Autodesk Inventor part; units mm, degrees
ref_plane "YZ Plane" through (0, 0, 0) normal (1, 0, 0) x (0, 1, 0)
ref_plane "XZ Plane" through (0, 0, 0) normal (0, 1, 0) x (-1, 0, 0)
ref_plane "XY Plane" through (0, 0, 0) normal (0, 0, 1) x (1, 0, 0)
sketch "Sketch2" plane through (0, 0, 0) normal (0, 0, 1) x (1, 0, 0)
  line L0 (150, -175) -> (-150, -175)
  line L1 (-150, -175) -> (-150, 175)
  line L2 (-150, 175) -> (150, 175)
  line L3 (150, 175) -> (150, -175)
  line L4 (150, -175) -> (-150, 175) construction
  line L5 (-150, -175) -> (150, 175) construction
  point P0 (0, 0)
  dimension "d0" = 300
  dimension "d1" = 350
extrude "Base" add sketch "Sketch2" along normal blind 300
shell "Shell1" thickness 5 removed faces 1 at (50, -58.3333, 300)
sketch "Sketch3" plane through (150, -175, 0) normal (1, 0, 0) x (0, 0, -1)
  circle A0 centre (-262.5, 27.5) radius 7.5
  line L0 (-300, 350) -> (-300, 0)
  line L1 (0, 0) -> (-300, 0)
  circle A1 centre (-237.5, 27.5) radius 7.5
  point P0 (0, 175)
  dimension "d5" = 15
  dimension "d9" = 37.5
  dimension "d10" = 27.5
  dimension "d13" = 25
extrude "Wire holes" cut sketch "Sketch3" against normal up to surface (5 mm away)
sketch "Sketch4" plane through (0, 0, 0) normal (0, 0, -1) x (-1, 0, 0)
  circle A0 centre (-96.967, -121.967) radius 25
  line L0 (-150, -175) -> (-96.967, -121.967) construction
  line L1 (-150, -175) -> (-75, -175) construction
  point P0 (0, 0)
  dimension "d20" = 50
  dimension "d21" = 75
  dimension "d22" = 45
extrude "Exhaust" cut sketch "Sketch4" against normal up to surface (5 mm away)
properties part number "mouse_SP_inner"
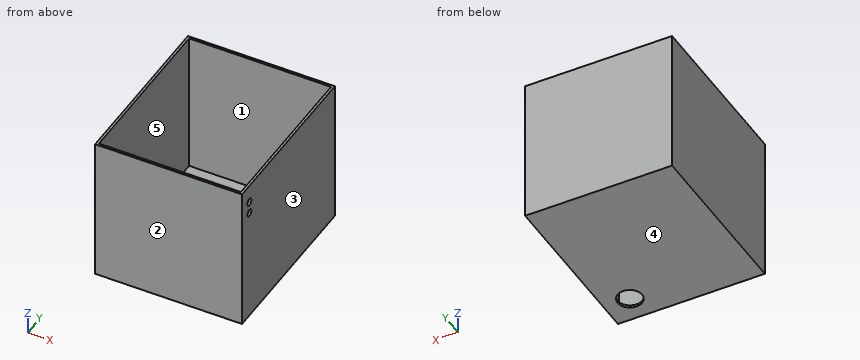
Geometry check sheet. Reference: the model listing, model coordinates, mm. Face numbers are marked on the shaded views. A direction names the side the tool comes from. Round coordinates to 2 decimals unless told otherwise and drop trailing zeros. Loops run counter-clockwise (first coordinate to the right, second up) from the corner with the lowest first, then second, coordinate; pieces in that order, holes last.
Item 1: Cross-section at A-A on x = -55. Record the boundary of the cut face in (y, z), then the cut area to 3 significant figures.
Item 2: Access from +Z, -Z, +X, -X, +Y, -Y to the whole of each face (thin tool, end or side, straight path). Record for the marked faces 1 and 2.
Item 3: Thickness scan on line 1 (Z direction, x = 148, y = -147); line 2 (X direction, y = 4, z = 17.5); line 3 (Y direction, x = 93, z = 92). Record the ranges inside material, lowest first.
Item 4: Mould release check, pull along X, two halves, no side actions. Record for the marked faces 3, 4 and 5: pulls with the +X half, pulls with the -X half, needs draft (parallel to the pull), parting line crosses it, or undercut.
Item 5: Gauge pin test, flat end, axial feed: pin 1 (2 mm diameter, centred on x = 40, y = 30.5, fed in from +Z). Record the tip position at first contact, or that the pin passes through.
Item 6: Cross-section at B-B on z = 21.5. Record the boundary of the cut face in (x, y).
Item 7: Cross-section at D-D on y = 132.5. Record the boundary of the cut face in (x, z).
Item 8: Cross-section at C-C on y = -135. Record the boundary of the cut face in (x, z), then the cut area to 3 significant figures.
Answer sheet:
1. outline: (-175, 0) - (175, 0) - (175, 300) - (170, 300) - (170, 5) - (-170, 5) - (-170, 300) - (-175, 300) - close
1. area: 4,700 mm2
2. face 1: +Z
2. face 2: +Z, -Z, +X, -X, -Y
3. line 1: z = 0 to 230.02, 244.98 to 255.02, 269.98 to 300
3. line 2: x = -150 to -145, 145 to 150
3. line 3: y = -175 to -170, 170 to 175
4. face 3: pulls with the +X half
4. face 4: needs draft
4. face 5: undercut
5. pin 1: stops at z = 5
6. outline: (-150, -175) - (150, -175) - (150, 175) - (-150, 175) - close; hole (-145, -170) - (145, -170) - (145, 170) - (-145, 170) - close
7. outline: (-150, 0) - (150, 0) - (150, 300) - (145, 300) - (145, 5) - (-145, 5) - (-145, 300) - (-150, 300) - close
8. outline: (-150, 0) - (75.63, 0) - (75.63, 5) - (-145, 5) - (-145, 300) - (-150, 300) - close; (118.3, 0) - (150, 0) - (150, 300) - (145, 300) - (145, 5) - (118.3, 5) - close
8. area: 4,240 mm2
